from build123d import *

# Parameters (mm, degrees)
SKETCH_AS_DRAWN_R                    = 9.6
EXTRUDE_DEPTH                        = 6
EXTRUDE_ONTO_SKETCH_ROLL_ANGLE       = 90
SKETCH001_AS_DRAWN_W                 = 150
SKETCH001_AS_DRAWN_H                 = 83
SKETCH001_AS_DRAWN_R                 = 5.5
EXTRUDE001_DEPTH                     = 10
EXTRUDE001_ONTO_SKETCH001_ROLL_ANGLE = 90


with BuildPart() as obj1:
    # Sketch as drawn → Extrude (new)
    with BuildSketch(Plane.XY):
        Circle(SKETCH_AS_DRAWN_R)
    extrude(amount=-EXTRUDE_DEPTH)


with BuildPart() as obj1_1:
    # Extrude onto Sketch roll: moved
    add(obj1.part.rotate(Axis((0, 0, 0), (1, 0, 0)), EXTRUDE_ONTO_SKETCH_ROLL_ANGLE))


with BuildPart() as obj1_2:
    # Extrude onto Sketch placement: moved
    add(obj1_1.part)


with BuildPart() as obj2:
    # Sketch001 as drawn → Extrude001 (new)
    with BuildSketch(Plane.XY):
        with Locations((-27.5, 23.5)):
            Rectangle(SKETCH001_AS_DRAWN_W, SKETCH001_AS_DRAWN_H)
        Circle(SKETCH001_AS_DRAWN_R, mode=Mode.SUBTRACT)
    extrude(amount=-EXTRUDE001_DEPTH)


with BuildPart() as obj2_1:
    # Extrude001 onto Sketch001 roll: moved
    add(obj2.part.rotate(Axis((0, 0, 0), (1, 0, 0)), EXTRUDE001_ONTO_SKETCH001_ROLL_ANGLE))


with BuildPart() as obj2_2:
    # Extrude001 onto Sketch001 placement: moved
    add(obj2_1.part)

    # Cut: cut obj1
    add(obj1_2.part, mode=Mode.SUBTRACT)


solid = obj2_2.part
Verification items for the finished model (mm, model axes). A direction names the side the tool comes from. Coordinates: 2 decimals unless noted, no trailing zeros. Loops run counter-clockwise (first coordinate to the right, second up) from the corner with the lowest first, then second, coordinate; pieces in that order, holes last. Notation, with made-up numbers: (-29, 43) -> (-13, 43) arc R20 cw to (-13, 59) -> close; hole circle Ø6 at (71.5, 29.25). An arc over 180 degrees is marked (long way). Answer as CSV lines item,"result".
1) Release check for a two-part mould opening along X. For faces 3 (the flat face through (-102.5, 5, 23)), 4 (the flat face through (47.5, 5, 23)), 5 (the cylindrical face through (-1.19, 7.97, -5.37)) record: +X half, -X half, draft (parallel to the pull), parting line (faces both ways), or undercut.
Found:
face 3,"-X half"
face 4,"+X half"
face 5,"undercut"
2) Cross-section at C-C, the plane y = 1.5. Record the cut outline in (x, z), then the cut area to 3 significant figures.
Found:
outline,"(-102.5, -18) -> (47.5, -18) -> (47.5, 65) -> (-102.5, 65) -> close; hole circle Ø19.2 at (0, 0)"
area,"12,200 mm2"
3) Cross-section at A-A, the plane x = 0. Record the cut outline in (y, z).
Found:
outline,"(0, -18) -> (10, -18) -> (10, -5.5) -> (6, -5.5) -> (6, -9.6) -> (0, -9.6) -> close; (0, 9.6) -> (6, 9.6) -> (6, 5.5) -> (10, 5.5) -> (10, 65) -> (0, 65) -> close"
4) Depth check by flat-ended pin: pin 1 (9 mm diameter, centred on x = 0, z = 0, fed in from +Y); pin 2 (6 mm diameter, centred on x = 1.5, z = 4.5, fed in from -Y). Enter the tip coordinate at first touch or a pass-through.
Found:
pin 1,"passes through"
pin 2,"stops at y = 6"
5) Tool access check on faces 1 (the flat face through (-29, 10, 24)), 2 (the flat face through (4, 6, -4)). Record the directions out of +Z, -Z, +X, -X, +Y, -Y that give a thin tool (end or side, any length) a straight path to the whole face; none if there is none.
Found:
face 1,"+Z, -Z, +X, -X, +Y"
face 2,"-Y"
6) Cross-section at B-B, the plane z = 0. Record the cut outline in (x, y).
Found:
outline,"(-102.5, 0) -> (-9.6, 0) -> (-9.6, 6) -> (-5.5, 6) -> (-5.5, 10) -> (-102.5, 10) -> close; (5.5, 6) -> (9.6, 6) -> (9.6, 0) -> (47.5, 0) -> (47.5, 10) -> (5.5, 10) -> close"
7) Thickness scan on L1, parallel to Z at x = 0, y = 4.5; L2, parallel to Z at x = 0, y = 7; L3, parallel to X at y = 4.75, z = -1. Record the ranges inside material, lowest first. Write a range as from..to.
Found:
L1,"z = -18..-9.6, 9.6..65"
L2,"z = -18..-5.5, 5.5..65"
L3,"x = -102.5..-9.55, 9.55..47.5"
